from build123d import *

# Parameters (mm, degrees)
SKETCH_1_R      = 15
SKETCH_1_R_2    = 1.65
EXTRUDE_1_DEPTH = 8
FILLET_1_R      = 1
EXTRUDE_2_DEPTH = 3


with BuildPart() as part:
    # 草图1 → 凸台-拉伸1 (new body)
    with BuildSketch(Plane.XY):
        Circle(SKETCH_1_R)
        Circle(SKETCH_1_R_2, mode=Mode.SUBTRACT)
        with Locations((0, 7)):
            Circle(SKETCH_1_R_2, mode=Mode.SUBTRACT)
        with Locations((7, 0)):
            Circle(SKETCH_1_R_2, mode=Mode.SUBTRACT)
        with Locations((0, -7)):
            Circle(SKETCH_1_R_2, mode=Mode.SUBTRACT)
        with Locations((-7, 0)):
            Circle(SKETCH_1_R_2, mode=Mode.SUBTRACT)
    extrude(amount=EXTRUDE_1_DEPTH)

    # 圆角1
    fillet_1_edges = [part.edges().sort_by_distance(p)[0] for p in [
        (-15, 0, 0),
    ]]
    fillet(fillet_1_edges, radius=FILLET_1_R)

    # 草图2 → 凸台-拉伸2 (add)
    with BuildSketch(Plane.XY.offset(8)):
        with BuildLine():
            ThreePointArc((-15, 0), (0, 15), (15, 0))
            Line((15, 0), (20, 0))
            ThreePointArc((20, 0), (0, 20), (-20, 0))
            Line((-20, 0), (-15, 0))
        make_face()
        with BuildLine():
            Line((20, 0), (15, 0))
            ThreePointArc((15, 0), (0, -15), (-15, 0))
            Line((-15, 0), (-20, 0))
            ThreePointArc((-20, 0), (0, -20), (20, 0))
        make_face()
        with BuildLine():
            Line((20, -75), (20, 0))
            ThreePointArc((20, 0), (0, -20), (-20, 0))
            Line((-20, 0), (-20, -75))
            Line((-20, -75), (20, -75))
        make_face()
    extrude(amount=-EXTRUDE_2_DEPTH)


solid = part.part
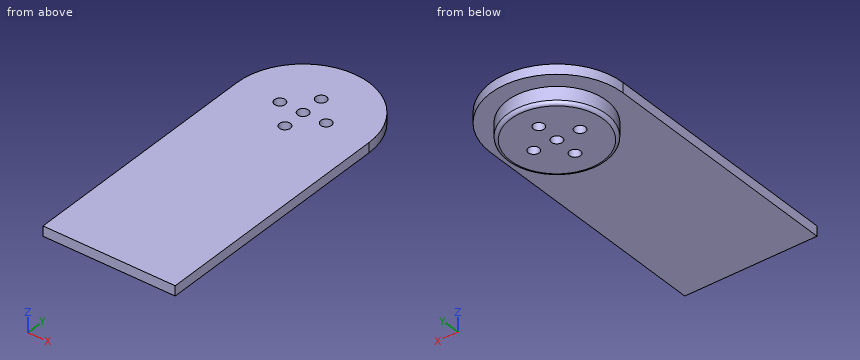
Model file for the job. Use its own axes, mm. Give positions to 0.01 mm unless a question says otherwise; leave off trailing zeros. Write each loop counter-clockwise with the first axis right and the second up, starting at its lowest first coordinate (ties: lowest second). Pieces come first, ordered by that corner, then holes. Notation, with made-up numbers: (12.5, 40) -> (64.5, 40) arc R7 ccw to (64.5, 47) -> close; hole circle Ø11 at (48, -8). An arc over 180 degrees is marked (long way). Write item = value, one per line.
(1) Slice it at C-C, the plane y = -20. Give the cut face in (x, z).
Determined:
outline = (-20, 5) -> (20, 5) -> (20, 8) -> (-20, 8) -> close
(2) Flat gauge pin, fed straight in: P1, Ø4, axis at x = 0, y = 7, coming from the +Z side. Where does the tip first touch, or does it go through?
Determined:
P1 = 8
(3) Slice it at A-A, the plane x = 0. Give the cut face in (y, z), then the cut area to 3 significant figures.
Determined:
outline = (-75, 5) -> (-15, 5) -> (-15, 1) arc R1 ccw to (-14, 0) -> (-8.65, 0) -> (-8.65, 8) -> (-75, 8) -> close; (-5.35, 0) -> (-1.65, 0) -> (-1.65, 8) -> (-5.35, 8) -> close; (1.65, 0) -> (5.35, 0) -> (5.35, 8) -> (1.65, 8) -> close; (8.65, 0) -> (14, 0) arc R1 ccw to (15, 1) -> (15, 5) -> (20, 5) -> (20, 8) -> (8.65, 8) -> close
area = 355 mm2
(4) Slice it at B-B, the plane z = 7. Give the cut face in (x, y), then the cut area to 3 significant figures.
Determined:
outline = (-20, -75) -> (20, -75) -> (20, 0) arc R20 ccw to (-20, 0) -> close; hole circle Ø3.3 at (-7, 0); hole circle Ø3.3 at (0, -7); hole circle Ø3.3 at (0, 0); hole circle Ø3.3 at (0, 7); hole circle Ø3.3 at (7, 0)
area = 3,590 mm2
(5) Slice it at D-D, the plane z = 3.25. Give the cut face in (x, y), then the cut area to 3 significant figures.
Determined:
outline = circle Ø30 at (0, 0); hole circle Ø3.3 at (-7, 0); hole circle Ø3.3 at (0, -7); hole circle Ø3.3 at (0, 0); hole circle Ø3.3 at (0, 7); hole circle Ø3.3 at (7, 0)
area = 664 mm2
(6) Probe line 1 along Y through (x, z) = (0, 2.5); line 2 along Y through (x, z) = (0, 6.25); line 3 along Z through (x, y) = (-8.5, -46). List the from-to ranges inside material, lowest first.
Determined:
line_1 = -15 to -8.65, -5.35 to -1.65, 1.65 to 5.35, 8.65 to 15
line_2 = -75 to -8.65, -5.35 to -1.65, 1.65 to 5.35, 8.65 to 20
line_3 = 5 to 8
